Read the model definition and answer for the solid it produces. Units are mm, in the model's axes. Face numbers are marked on the shaded views. A direction names the side the tool comes from. Give positions to 0.01 mm unless a question says otherwise; leave off trailing zeros. Order: outer loops, then holes, each group sorted by start corner. A loop starts at its lowest first (then second) coordinate and runs counter-clockwise, first axis right, second up.
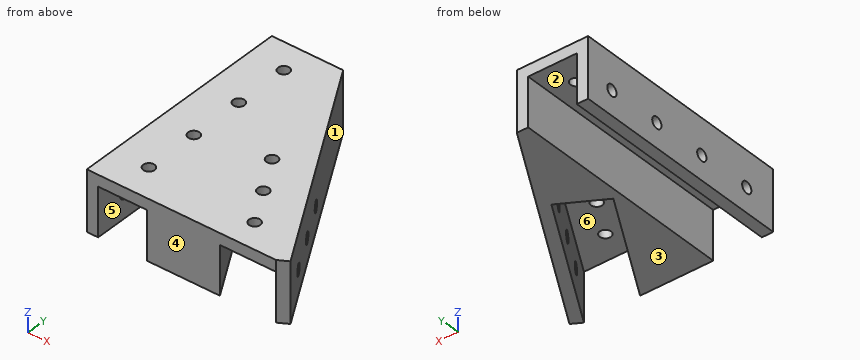
```python
from build123d import *

# Parameters (mm, degrees)
BOSS_EXTRUDE1_DEPTH = 18.5
SKETCH2_W           = 15
SKETCH2_H           = 69.980762113
CUT_EXTRUDE1_DEPTH  = 15
SKETCH3_R           = 1.75
CUT_EXTRUDE2_DEPTH  = 3.5
SKETCH4_R           = 1.75
CUT_EXTRUDE3_DEPTH  = 4
SKETCH5_R           = 1.75
CUT_EXTRUDE4_DEPTH  = 4
CUT_EXTRUDE5_DEPTH  = 19


with BuildPart() as part:
    # Sketch1 → Boss-Extrude1 (new body)
    with BuildSketch(Plane.XY):
        Polygon((7.85498998, 37.469557102), (48.258401824, -32.511205011), (7.85498998, -32.511205011), (-14.14501002, -32.511205011), (-14.14501002, 37.469557102), align=None)
    extrude(amount=BOSS_EXTRUDE1_DEPTH)

    # Sketch2 → Cut-Extrude1 (cut)
    with BuildSketch(Plane.XY):
        with Locations((-3.14501002, 2.479176046)):
            Rectangle(SKETCH2_W, SKETCH2_H)
        Polygon((44.21694994, -32.511205011), (19.886822921, 9.62981114), (6.896441864, 2.12981114), (26.896441864, -32.511205011), align=None)
    extrude(amount=CUT_EXTRUDE1_DEPTH, mode=Mode.SUBTRACT)

    # Sketch3 → Cut-Extrude2 (cut)
    with BuildSketch(Plane(origin=(22.116036645, 12.76869971, 0), x_dir=(0, 0, -1), z_dir=(0.8660254037844378, 0.5000000000000016, 0))):
        with Locations(Location((-7.5, -38.284730359, 0), (0, 0, 90))):
            Circle(SKETCH3_R)
        with Locations(Location((-7.5, -25.284730359, 0), (0, 0, 90))):
            Circle(SKETCH3_R)
        with Locations(Location((-7.5, -12.284730359, 0), (0, 0, 90))):
            Circle(SKETCH3_R)
    extrude(amount=-CUT_EXTRUDE2_DEPTH, mode=Mode.SUBTRACT)

    # Sketch4 → Cut-Extrude3 (cut)
    with BuildSketch(Plane(origin=(0, 0, 18.5), x_dir=(-1, 0, 0), z_dir=(0, 0, -1))):
        with Locations(Location((-30.556695902, -23.850950973, 0), (0, 0, 180))):
            Circle(SKETCH4_R)
        with Locations(Location((-24.056695902, -12.592620724, 0), (0, 0, 180))):
            Circle(SKETCH4_R)
        with Locations(Location((-17.556695902, -1.334290475, 0), (0, 0, 180))):
            Circle(SKETCH4_R)
        with Locations(Location((3.14501002, -5.511205011, 0), (0, 0, 180))):
            Circle(SKETCH4_R)
        with Locations(Location((3.14501002, 11.488794989, 0), (0, 0, 180))):
            Circle(SKETCH4_R)
        with Locations(Location((3.14501002, 28.488794989, 0), (0, 0, 180))):
            Circle(SKETCH4_R)
        with Locations(Location((3.14501002, -22.511205011, 0), (0, 0, 180))):
            Circle(SKETCH4_R)
    extrude(amount=CUT_EXTRUDE3_DEPTH, mode=Mode.SUBTRACT)

    # Sketch5 → Cut-Extrude4 (cut)
    with BuildSketch(Plane.ZY.offset(14.14501002)):
        with Locations(Location((7.5, -22.511205011, 0), (0, 0, 270))):
            Circle(SKETCH5_R)
        with Locations(Location((7.5, -5.511205011, 0), (0, 0, 270))):
            Circle(SKETCH5_R)
        with Locations(Location((7.5, 11.488794989, 0), (0, 0, 270))):
            Circle(SKETCH5_R)
        with Locations(Location((7.5, 28.488794989, 0), (0, 0, 270))):
            Circle(SKETCH5_R)
    extrude(amount=-CUT_EXTRUDE4_DEPTH, mode=Mode.SUBTRACT)

    # Sketch6 → Cut-Extrude5 (cut)
    with BuildSketch(Plane.XY.offset(18.5)):
        Polygon((44.21694994, -32.511205011), (47.248038853, -30.761205011), (48.258401824, -32.511205011), align=None)
    extrude(amount=-CUT_EXTRUDE5_DEPTH, mode=Mode.SUBTRACT)


solid = part.part
```
1) Consider L1, parallel to X at y = -28.5, z = 14.5; L2, parallel to X at y = -8.5, z = 3; L3, parallel to Z at x = 20, y = -14. Determine where each line is inside the solid, lowest interval first.
Final values:
L1: x = -14.15 to -10.65, 4.35 to 24.58, 41.9 to 45.94
L2: x = -14.15 to -10.65, 4.35 to 13.03, 30.35 to 34.4
L3: z = 15 to 18.5
2) The part is cut by section C-C on x = 21. Determine the outline of the cut face in (y, z).
Final values:
outline: (-32.51, 0) - (-22.3, 0) - (-22.3, 15) - (7.7, 15) - (7.7, 0) - (14.7, 0) - (14.7, 18.5) - (-32.51, 18.5) - close
3) For a pull along X with two mould halves and no side action, classify the marked faces 1, 2 and 3 as released by +X, released by -X, zero draft, split by the parting line, or undercut.
Final values:
face 1: released by +X
face 2: undercut
face 3: zero draft
4) Given pin 1 (2 mm diameter, centred on y = -5.51, z = 7.5, fed in from -X) (3 decimals); pin 2 (1.5 mm diameter, centred on x = 0, y = 4, fed in from -Z); pin 3 (4.5 mm diameter, centred on y = 10, z = 4, fed in from +X), each flat-ended and moving along its own axis, determine where each tip first touches the part or whether it passes through.
Final values:
pin 1: stops at x = 4.355
pin 2: stops at z = 15
pin 3: stops at x = 25.01
5) The part is cut by section D-D on z = 7.5. Count the separate pieces of the cut face and the enclosed holes in it, and give its area (3 significant figures).
Final values:
separate pieces: 9
enclosed holes: 0
area: 1,150 mm2
6) A tool of negligible diameter and unlimited length cuts with its end or side. For the marked faces 4, 5 and 6, from which of +Z, -Z, +X, -X, +Y, -Y can it reach the whole face along a straight path? Write none if from no direction.
Final values:
face 4: +Z, -Z, +X, -X, -Y
face 5: -Z, +Y, -Y
face 6: -Z
7) The part is cut by section A-A on z = 11.75. Determine the outline of the cut face in (x, y), and give its area (3 significant figures).
Final values:
outline: (-14.15, -32.51) - (-10.65, -32.51) - (-10.65, 37.47) - (-14.15, 37.47) - close; (4.35, -32.51) - (26.9, -32.51) - (6.9, 2.13) - (19.89, 9.63) - (44.22, -32.51) - (47.25, -30.76) - (7.85, 37.47) - (4.35, 37.47) - close
area: 1,240 mm2
8) The part is cut by section B-B on y = 27.5. Determine the outline of the cut face in (x, z).
Final values:
outline: (-14.15, 0) - (-10.65, 0) - (-10.65, 6.06) - (-14.15, 6.06) - close; (-14.15, 8.94) - (-10.65, 8.94) - (-10.65, 15) - (-4.59, 15) - (-4.59, 18.5) - (-14.15, 18.5) - close; (-1.7, 15) - (4.35, 15) - (4.35, 0) - (13.61, 0) - (13.61, 18.5) - (-1.7, 18.5) - close
